Source: CAD feature listing. Evaluate the final solid. Frame: model axes, mm. Coordinates: 2 decimals unless noted, no trailing zeros.
Item 1: Contact query for flat-ended pins moving along their axis: P1, Ø4, axis at x = -11, y = -18, coming from the +Z side; P2, Ø2, axis at x = -23.5, z = 3, coming from the -Y side. Output: stop coordinate, or through.
Item 2: Section A-A on z = 2. State how many separate pieces and enclosed holes the cut face has, then the cut area to 3 significant figures.
Item 3: Ray query, line 1 (X direction, y = 16.5, z = 4.25); line 2 (X direction, y = 33.5, z = 7); line 3 (Y direction, x = 27, z = 1.25). Return the intervals inside material, ascending.
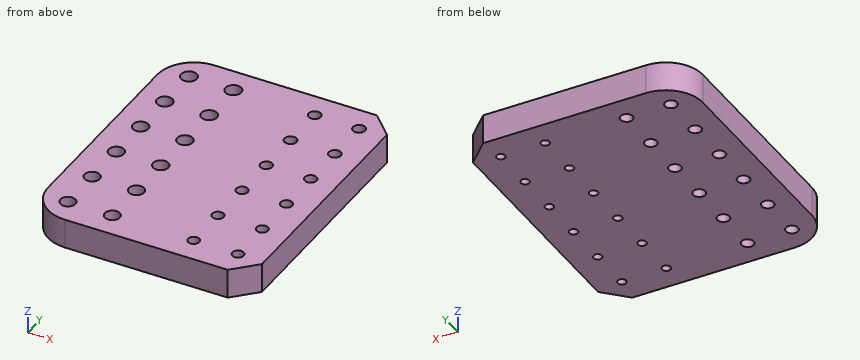
from build123d import *

# Parameters (mm, degrees)
SKETCH1_W           = 60
SKETCH1_H           = 74
BOSS_EXTRUDE1_DEPTH = 12
SKETCH3_R           = 1.65
SKETCH3_R_2         = 1.15
CUT_EXTRUDE1_DEPTH  = 50.122296363
CHAMFER1_SIZE       = 6
FILLET1_R           = 10
SKETCH4_R           = 2.9
SKETCH4_R_2         = 2.4
CUT_EXTRUDE2_DEPTH  = 4
SKETCH6_R           = 2.15
SKETCH6_R_2         = 2.125
SKETCH6_R_3         = 2.1
SKETCH6_R_4         = 2.075
SKETCH6_R_5         = 2.05
SKETCH6_R_6         = 2.025
SKETCH6_R_7         = 1.525
SKETCH6_R_8         = 1.55
SKETCH6_R_9         = 1.575
SKETCH6_R_10        = 1.6
SKETCH6_R_11        = 1.625
SKETCH6_R_12        = 1.65
CUT_EXTRUDE3_DEPTH  = 3.1
SKETCH8_W           = 4
SKETCH8_H           = 74
CUT_EXTRUDE4_DEPTH  = 72.505244563


with BuildPart() as part:
    # Sketch1 → Boss-Extrude1 (new body)
    with BuildSketch(Plane.XY):
        Rectangle(SKETCH1_W, SKETCH1_H)
    extrude(amount=BOSS_EXTRUDE1_DEPTH)

    # Sketch3 → Cut-Extrude1 (cut, through all)
    with BuildSketch(Plane.XY.offset(12)):
        with Locations((-23, -30)):
            Circle(SKETCH3_R)
        with Locations((23, -30)):
            Circle(SKETCH3_R_2)
        with Locations((-11, -30)):
            Circle(SKETCH3_R)
        with Locations((-11, -18)):
            Circle(SKETCH3_R)
        with Locations((-11, -6)):
            Circle(SKETCH3_R)
        with Locations((-11, 6)):
            Circle(SKETCH3_R)
        with Locations((-23, -18)):
            Circle(SKETCH3_R)
        with Locations((-23, -6)):
            Circle(SKETCH3_R)
        with Locations((-23, 6)):
            Circle(SKETCH3_R)
        with Locations((11, -30)):
            Circle(SKETCH3_R_2)
        with Locations((11, -18)):
            Circle(SKETCH3_R_2)
        with Locations((11, -6)):
            Circle(SKETCH3_R_2)
        with Locations((11, 6)):
            Circle(SKETCH3_R_2)
        with Locations((23, -18)):
            Circle(SKETCH3_R_2)
        with Locations((23, -6)):
            Circle(SKETCH3_R_2)
        with Locations((23, 6)):
            Circle(SKETCH3_R_2)
        with Locations((-23, 18)):
            Circle(SKETCH3_R)
        with Locations((-11, 18)):
            Circle(SKETCH3_R)
        with Locations((-23, 30)):
            Circle(SKETCH3_R)
        with Locations((-11, 30)):
            Circle(SKETCH3_R)
        with Locations((23, 18)):
            Circle(SKETCH3_R_2)
        with Locations((11, 18)):
            Circle(SKETCH3_R_2)
        with Locations((23, 30)):
            Circle(SKETCH3_R_2)
        with Locations((11, 30)):
            Circle(SKETCH3_R_2)
    extrude(amount=-CUT_EXTRUDE1_DEPTH, mode=Mode.SUBTRACT)

    # Chamfer1
    chamfer1_edges = [part.edges().sort_by_distance(p)[0] for p in [
        (30, 37, 6),
        (30, -37, 6),
    ]]
    chamfer(chamfer1_edges, length=CHAMFER1_SIZE)

    # Fillet1
    fillet1_edges = [part.edges().sort_by_distance(p)[0] for p in [
        (-30, 37, 6),
        (-30, -37, 6),
    ]]
    fillet(fillet1_edges, radius=FILLET1_R)

    # Sketch4 → Cut-Extrude2 (cut)
    with BuildSketch(Plane.XY.offset(12)):
        with Locations((-23, -30)):
            Circle(SKETCH4_R)
        with Locations((-11, -30)):
            Circle(SKETCH4_R)
        with Locations((-11, -18)):
            Circle(SKETCH4_R)
        with Locations((-11, -6)):
            Circle(SKETCH4_R)
        with Locations((-11, 6)):
            Circle(SKETCH4_R)
        with Locations((-23, -18)):
            Circle(SKETCH4_R)
        with Locations((-23, -6)):
            Circle(SKETCH4_R)
        with Locations((-23, 6)):
            Circle(SKETCH4_R)
        with Locations((11, -30)):
            Circle(SKETCH4_R_2)
        with Locations((23, -30)):
            Circle(SKETCH4_R_2)
        with Locations((23, -18)):
            Circle(SKETCH4_R_2)
        with Locations((23, -6)):
            Circle(SKETCH4_R_2)
        with Locations((23, 6)):
            Circle(SKETCH4_R_2)
        with Locations((11, -18)):
            Circle(SKETCH4_R_2)
        with Locations((11, -6)):
            Circle(SKETCH4_R_2)
        with Locations((11, 6)):
            Circle(SKETCH4_R_2)
        with Locations((-23, 18)):
            Circle(SKETCH4_R)
        with Locations((-11, 18)):
            Circle(SKETCH4_R)
        with Locations((-23, 30)):
            Circle(SKETCH4_R)
        with Locations((-11, 30)):
            Circle(SKETCH4_R)
        with Locations((11, 18)):
            Circle(SKETCH4_R_2)
        with Locations((23, 18)):
            Circle(SKETCH4_R_2)
        with Locations((11, 30)):
            Circle(SKETCH4_R_2)
        with Locations((23, 30)):
            Circle(SKETCH4_R_2)
    extrude(amount=-CUT_EXTRUDE2_DEPTH, mode=Mode.SUBTRACT)

    # Sketch6 → Cut-Extrude3 (cut)
    with BuildSketch(Plane.XY.offset(8)):
        with Locations((-23, 30)):
            Circle(SKETCH6_R)
        with Locations((-23, 18)):
            Circle(SKETCH6_R_2)
        with Locations((-23, 6)):
            Circle(SKETCH6_R_3)
        with Locations((-23, -6)):
            Circle(SKETCH6_R_4)
        with Locations((-23, -18)):
            Circle(SKETCH6_R_5)
        with Locations((-23, -30)):
            Circle(SKETCH6_R_6)
        with Locations((-11, 30)):
            Circle(SKETCH6_R)
        with Locations((11, -30)):
            Circle(SKETCH6_R_7)
        with Locations((11, -18)):
            Circle(SKETCH6_R_8)
        with Locations((11, -6)):
            Circle(SKETCH6_R_9)
        with Locations((11, 6)):
            Circle(SKETCH6_R_10)
        with Locations((11, 18)):
            Circle(SKETCH6_R_11)
        with Locations((11, 30)):
            Circle(SKETCH6_R_12)
        with Locations((-11, 18)):
            Circle(SKETCH6_R_2)
        with Locations((-11, 6)):
            Circle(SKETCH6_R_3)
        with Locations((-11, -6)):
            Circle(SKETCH6_R_4)
        with Locations((-11, -18)):
            Circle(SKETCH6_R_5)
        with Locations((-11, -30)):
            Circle(SKETCH6_R_6)
        with Locations((23, -30)):
            Circle(SKETCH6_R_7)
        with Locations((23, -18)):
            Circle(SKETCH6_R_8)
        with Locations((23, -6)):
            Circle(SKETCH6_R_9)
        with Locations((23, 6)):
            Circle(SKETCH6_R_10)
        with Locations((23, 18)):
            Circle(SKETCH6_R_11)
        with Locations((23, 30)):
            Circle(SKETCH6_R_12)
    extrude(amount=-CUT_EXTRUDE3_DEPTH, mode=Mode.SUBTRACT)

    # Sketch8 → Cut-Extrude4 (cut, through all)
    with BuildSketch(Plane.ZY.offset(30)):
        with Locations((10, 0)):
            Rectangle(SKETCH8_W, SKETCH8_H)
    extrude(amount=-CUT_EXTRUDE4_DEPTH, mode=Mode.SUBTRACT)


solid = part.part
Answer list:
1. P1: stops at z = 4.9
1. P2: stops at y = -36.68
2. separate pieces: 1
2. enclosed holes: 24
2. area: 4,210 mm2
3. line 1: x = -30 to -23.69, -22.31 to -11.69, -10.31 to 30
3. line 2: x = -27.6 to 27.5
3. line 3: y = -34 to 34
